Input: dimensioned drawing with shaded views. Units: mm. Origin: part minimum x, y, z. A direction names the side the tool comes from. Give positions to 0.01 mm unless a question says otherwise; leave off trailing zeros. Loops run counter-clockwise (first coordinate to the right, second up) from the corner with the lowest first, then second, coordinate; pieces in that order, holes last. Notation, with made-up numbers: M -29,10 L 5,10 A13 cw 5,25 Z; hole C 27,-4 d9. An arc over 180 degrees is marked long. Use CSV: the item, a comma, the result in double quotes. Start each with the question number.
Q1. Reachability of the marked faces 4 and 5 from +Z, -Z, +X, -X, +Y, -Y: full face, straight path, thin tool, end or side. Return the list, or none.
Q2. Material intervals for line 1 along Z through (x, y) = (7, 0.95); line 2 along Z through (x, y) = (7, 4.5); line 3 along Y through (x, z) = (6.25, 3.5), sorted ascending.
Q3. Section D-D, the plane y = 6.75. Output: boundary loops of the cut face in (x, z), plus the area to 3 significant figures.
Q4. Section A-A, the plane z = 7. Output: boundary loops of the cut face in (x, y), plus the area to 3 significant figures.
Q5. Section B-B, the plane x = 7. Output: boundary loops of the cut face in (y, z).
Q6. Section C-C, the plane y = 2.25. Output: boundary loops of the cut face in (x, z).
Q7. Pull-direction query (X, two-part tool) for the marked faces 1, 2 and 3; classes: released by +X, released by -X, zero draft, split by the parting line, or undercut.
Q8. Pin query (flat end, axial travel): pin 1 (1 mm diameter, centred on x = 8.5, z = 7, fed in from -Y); pin 2 (2 mm diameter, centred on y = 5.5, z = 3.5, fed in from +X); pin 3 (1 mm diameter, centred on y = 3.5, z = 5, fed in from +X). Return the tip coordinate at first contact, or that it passes through.
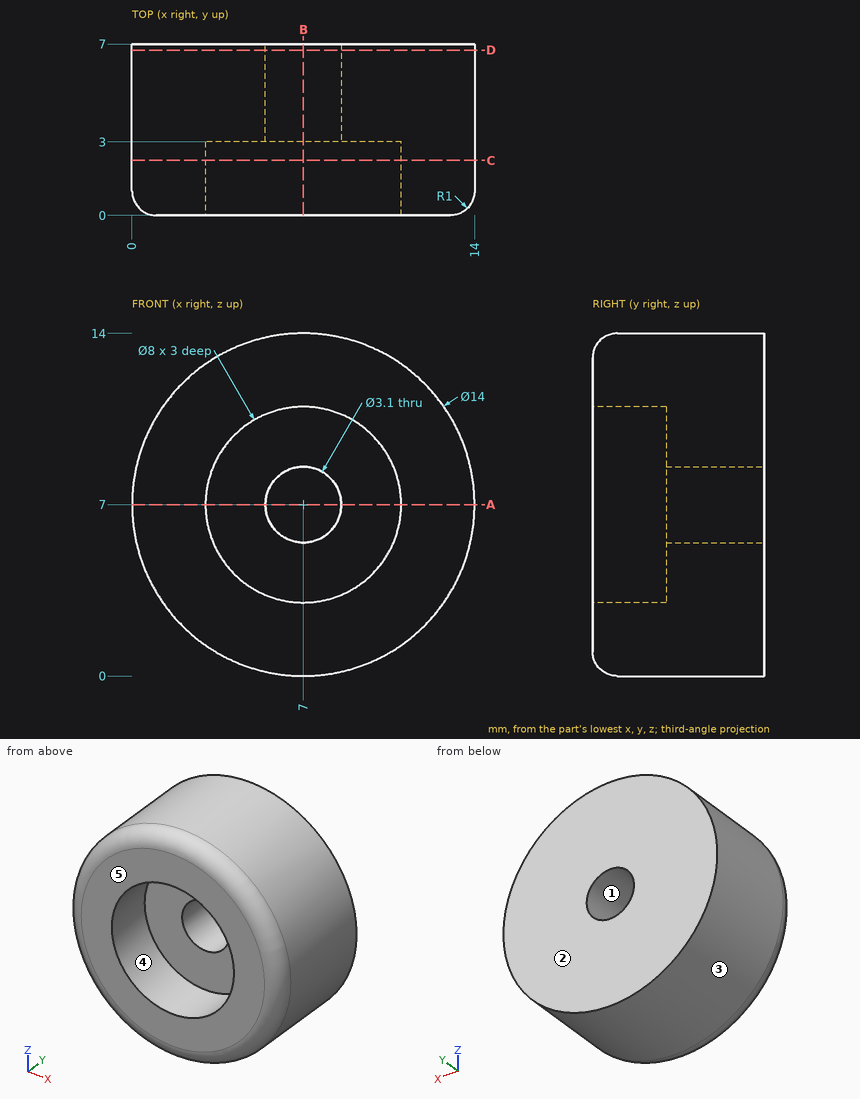
A:
1,face 4,"-Y"
1,face 5,"+Z, -Z, +X, -X, -Y"
2,line 1,"0 to 3, 11 to 14"
2,line 2,"0 to 5.45, 8.55 to 14"
2,line 3,"3 to 7"
3,outline,"C 7,7 d14; hole C 7,7 d3.1"
3,area,"146 mm^2"
4,outline,"M 0,1 A1 ccw 1,0 L 3,0 L 3,3 L 5.45,3 L 5.45,7 L 0,7 Z; M 8.55,3 L 11,3 L 11,0 L 13,0 A1 ccw 14,1 L 14,7 L 8.55,7 Z"
4,area,"61.2 mm^2"
5,outline,"M 0,1 A1 ccw 1,0 L 7,0 L 7,5.45 L 3,5.45 L 3,3 L 0,3 Z; M 0,11 L 3,11 L 3,8.55 L 7,8.55 L 7,14 L 1,14 A1 ccw 0,13 Z"
6,outline,"C 7,7 d14; hole C 7,7 d8"
7,face 1,"undercut"
7,face 2,"zero draft"
7,face 3,"split by the parting line"
8,pin 1,"y = 3"
8,pin 2,"x = 13.54"
8,pin 3,"x = 13.84"
